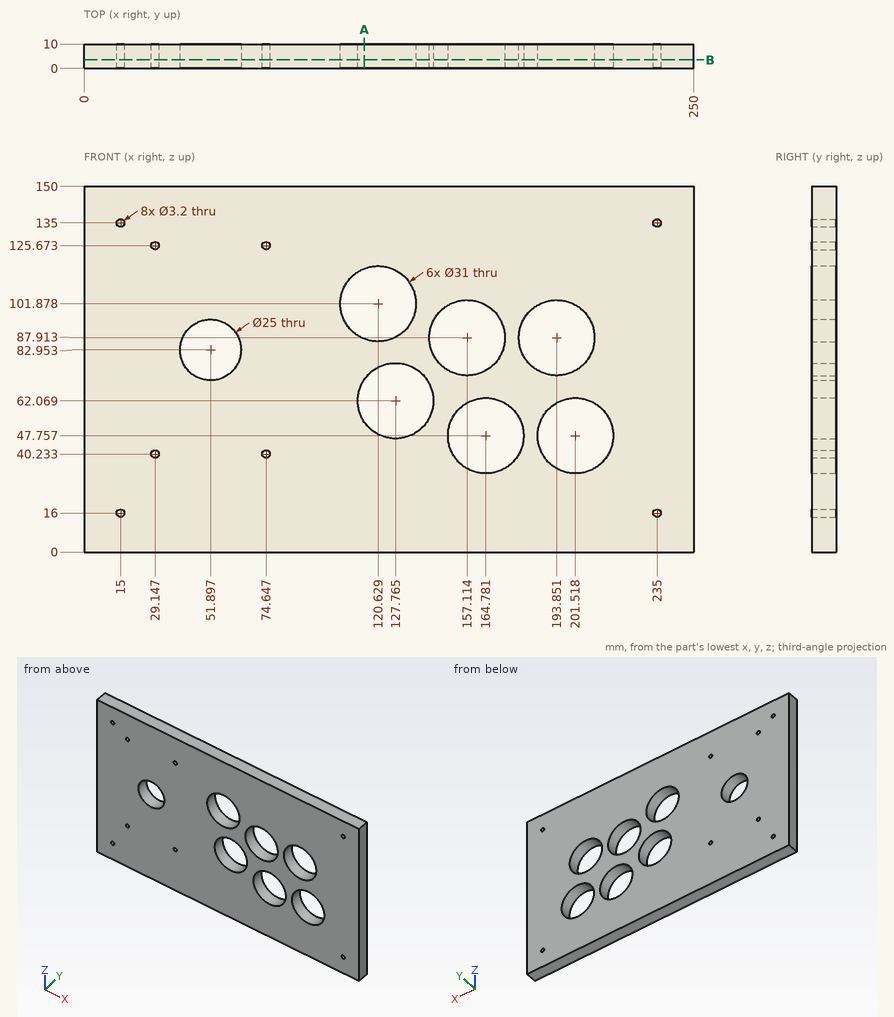
Source: three-view drawing plus pictorial views. Frame: mm from the lowest corner of the part. Coordinates: 2 decimals unless noted, no trailing zeros. Loops run counter-clockwise (first coordinate to the right, second up) from the corner with the lowest first, then second, coordinate; pieces in that order, holes last. Notation, with made-up numbers: (41.5, -7.75) - (70.5, -7.75) arc R25 cw to (70.5, 21.25) - close; hole circle Ø2 at (59, 68.5). An arc over 180 degrees is marked (long way). Answer in a Markdown table with one row per item. Add a question column.
Item 1: Section query A-A on x = 115. Return the cut outline in (y, z), then the cut area to 3 significant figures.
Item 2: Line query: line 1 along X through (y, z) = (7, 16); line 2 along Z through (x, y) = (168, 3.5) (1 decimal); line 3 along Z through (x, y) = (169, 8) (1 decimal). Output: solid intervals per line, ascending. Write a range as [from, to].
Item 3: Section query B-B on y = 3.5. State how many separate pieces and enclosed holes the cut face has, then the cut area to 3 significant figures.
Recorded:
| question | item | result |
|---|---|---|
| 1 | outline | (0, 0) - (10, 0) - (10, 53.28) - (0, 53.28) - close; (0, 70.86) - (10, 70.86) - (10, 87.44) - (0, 87.44) - close; (0, 116.32) - (10, 116.32) - (10, 150) - (0, 150) - close |
| 1 | area | 1,040 mm^2 |
| 2 | line 1 | [0, 13.4], [16.6, 233.4], [236.6, 250] |
| 2 | line 2 | [0, 32.6], [62.9, 76.9], [98.9, 150] |
| 2 | line 3 | [0, 32.8], [62.7, 78], [97.9, 150] |
| 3 | separate pieces | 1 |
| 3 | enclosed holes | 15 |
| 3 | area | 32,400 mm^2 |
